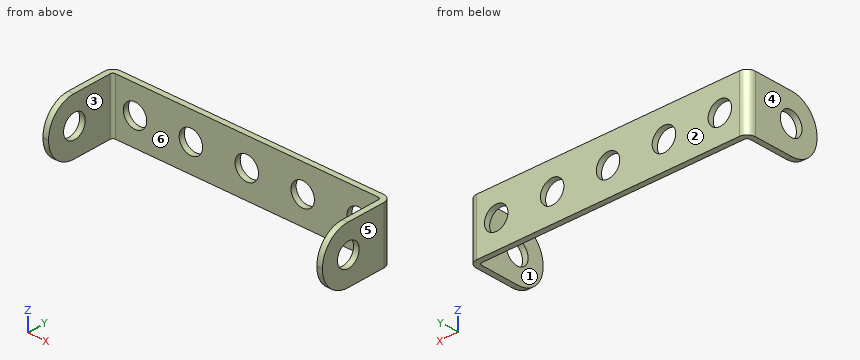
```python
from build123d import *

# Parameters (mm, degrees)
PAD_DEPTH       = 10
FILLET_R        = 4.9
FILLET001_R     = 4.9
FILLET002_R     = 4.9
FILLET003_R     = 4.9
SKETCH001_R     = 2.1
POCKET_DEPTH    = 50.001
SKETCH002_R     = 2.1
POCKET001_DEPTH = 13.401


with BuildPart() as part:
    # Sketch → Pad (new body)
    with BuildSketch(Plane.XY):
        with BuildLine():
            Line((0, 0), (0, 11.9))
            ThreePointArc((1.5, 13.4), (0.43934, 12.96066), (0, 11.9))
            Line((1.5, 13.4), (48.5, 13.4))
            ThreePointArc((50, 11.9), (49.56066, 12.96066), (48.5, 13.4))
            Line((50, 11.9), (50, 0))
            Line((49, 0), (50, 0))
            Line((49, 11.9), (49, 0))
            ThreePointArc((49, 11.9), (48.853553, 12.253553), (48.5, 12.4))
            Line((1.5, 12.4), (48.5, 12.4))
            ThreePointArc((1.5, 12.4), (1.146447, 12.253553), (1, 11.9))
            Line((1, 0), (1, 11.9))
            Line((0, 0), (1, 0))
        make_face()
    extrude(amount=PAD_DEPTH)

    # Fillet
    fillet_edges = [part.edges().sort_by_distance(p)[0] for p in [
        (49.5, 0, 0),
    ]]
    fillet(fillet_edges, radius=FILLET_R)

    # Fillet001
    fillet001_edges = [part.edges().sort_by_distance(p)[0] for p in [
        (0.5, 0, 0),
    ]]
    fillet(fillet001_edges, radius=FILLET001_R)

    # Fillet002
    fillet002_edges = [part.edges().sort_by_distance(p)[0] for p in [
        (49.5, 0, 10),
    ]]
    fillet(fillet002_edges, radius=FILLET002_R)

    # Fillet003
    fillet003_edges = [part.edges().sort_by_distance(p)[0] for p in [
        (0.5, 0, 10),
    ]]
    fillet(fillet003_edges, radius=FILLET003_R)

    # Sketch001 → Pocket (cut, through all)
    with BuildSketch(Plane(origin=(0, 0, 0), x_dir=(0, -1, 0), z_dir=(-1, 0, 0))):
        with Locations((-5, 5)):
            Circle(SKETCH001_R)
    extrude(amount=-POCKET_DEPTH, mode=Mode.SUBTRACT)

    # Sketch002 → Pocket001 (cut, through all)
    with BuildSketch(Plane(origin=(0, 13.4, 0), x_dir=(-1, 0, 0), z_dir=(0, 1, 0))):
        with Locations((-5, 5)):
            Circle(SKETCH002_R)
        with Locations((-15, 5)):
            Circle(SKETCH002_R)
        with Locations((-25, 5)):
            Circle(SKETCH002_R)
        with Locations((-35, 5)):
            Circle(SKETCH002_R)
        with Locations((-45, 5)):
            Circle(SKETCH002_R)
    extrude(amount=-POCKET001_DEPTH, mode=Mode.SUBTRACT)


solid = part.part
```
Part model, mm, in its own coordinate system. Face numbers are marked on the shaded views. A direction names the side the tool comes from. Round coordinates to 2 decimals unless told otherwise and drop trailing zeros. Order: outer loops, then holes, each group sorted by start corner. A loop starts at its lowest first (then second) coordinate and runs counter-clockwise, first axis right, second up. Notation, with made-up numbers: M 64,-30 L 89,-30 A19 cw 89,-18 Z; hole C -34.75,35.5 d4. An arc over 180 degrees is marked long. Put each result on its own line as item: value. Start each with the question number.
1. Tool access for the marked faces 1 and 2: list every direction of +Z, -Z, +X, -X, +Y, -Y with a clear straight run to the whole face (end or side of a thin tool).
2. Slice it at C-C on y = 3.75. List the corners of the cut face in (x, z), then the cut area to 3 significant figures.
3. Slice it at D-D on z = 3.75. State how many separate pieces and enclosed holes the cut face has, then the cut area to 3 significant figures.
4. Slice it at A-A on x = 45. List the corners of the cut face in (y, z), then the cut area to 3 significant figures.
5. Two-plate mould, pull along X, no slides. Class the marked faces 3, 4, 5 and 6: +X half, -X half, draft (parallel to the pull), parting line (faces both ways), or undercut.
6. Drill centre lines: probe 1 along Z at (x, y) = (5, 12.9); probe 2 along X at (y, z) = (6.5, 7.75); probe 3 along Y at (x, z) = (13, 6.5). Where is each one in solid material? Low to high. Write a range as [from, to].
7. Slice it at B-B on y = 8.5. List the corners of the cut face in (x, z), then the cut area to 3 significant figures.
8. Drop flat-ended pins along their axis: pin 1 (2.5 mm diameter, centred on x = 15, z = 5, fed in from -Y); pin 2 (1 mm diameter, centred on x = 11.5, z = 2.5, fed in from -Y). Give the stop position or say it passes through.
Findings:
1. face 1: +Z, -Z, -Y
1. face 2: +Z, -Z, +X, -X, +Y
2. outline: M 0,0.14 L 1,0.14 L 1,3.31 L 0,3.31 Z; M 0,6.69 L 1,6.69 L 1,9.86 L 0,9.86 Z; M 49,0.14 L 50,0.14 L 50,3.31 L 49,3.31 Z; M 49,6.69 L 50,6.69 L 50,9.86 L 49,9.86 Z
2. area: 12.7 mm2
3. separate pieces: 8
3. enclosed holes: 0
3. area: 50.0 mm2
4. outline: M 12.4,0 L 13.4,0 L 13.4,2.9 L 12.4,2.9 Z; M 12.4,7.1 L 13.4,7.1 L 13.4,10 L 12.4,10 Z
4. area: 5.80 mm2
5. face 3: undercut
5. face 4: -X half
5. face 5: +X half
5. face 6: undercut
6. probe 1: [0, 2.9], [7.1, 10]
6. probe 2: [0, 1], [49, 50]
6. probe 3: [12.4, 13.4]
7. outline: M 0,0 L 1,0 L 1,10 L 0,10 Z; M 49,0 L 50,0 L 50,10 L 49,10 Z
7. area: 20.0 mm2
8. pin 1: through
8. pin 2: y = 12.4
